For this review, take the finished solid that the model builds, in its own axes (mm). Round coordinates to 2 decimals unless told otherwise and drop trailing zeros. Order: outer loops, then holes, each group sorted by start corner. A loop starts at its lowest first (then second) coordinate and runs counter-clockwise, first axis right, second up. Notation, with made-up numbers: (32.25, 80.25) -> (53.25, 80.25) arc R20 cw to (53.25, 91.25) -> close; hole circle Ø2 at (-17.75, -9). An arc over 180 degrees is marked (long way). Put each result on its own line as item: value. Start each with the question number.
```python
from build123d import *

# Parameters (mm, degrees)
SKETCH1_W                = 80
SKETCH1_H                = 124.77
SKETCH1_R                = 5.5
BOSS_EXTRUDE1_DEPTH      = 6
F_5_0_5_DIAMETER_HOLE1_D = 5
M5X0_8_TAPPED_HOLE1_D    = 4.2
CHAMFER1_SIZE            = 2.5


with BuildPart() as part:
    # Sketch1 → Boss-Extrude1 (new body)
    with BuildSketch(Plane.XY):
        with Locations((40, 62.385)):
            Rectangle(SKETCH1_W, SKETCH1_H)
        with Locations((40, 17.57)):
            Circle(SKETCH1_R, mode=Mode.SUBTRACT)
        with BuildLine():
            Line((59.1, 94.58), (59.1, 86.58))
            ThreePointArc((59.1, 86.58), (40, 67.48), (20.9, 86.58))
            Line((20.9, 86.58), (20.9, 94.58))
            ThreePointArc((20.9, 94.58), (40, 113.68), (59.1, 94.58))
        make_face(mode=Mode.SUBTRACT)
        with BuildLine():
            Line((18.97, 118.15), (18.97, 111.15))
            ThreePointArc((18.97, 111.15), (16.43, 108.61), (13.89, 111.15))
            Line((13.89, 111.15), (13.89, 118.15))
            ThreePointArc((13.89, 118.15), (16.43, 120.69), (18.97, 118.15))
        make_face(mode=Mode.SUBTRACT)
        with BuildLine():
            Line((61.03, 118.15), (61.03, 111.15))
            ThreePointArc((61.03, 111.15), (63.57, 108.61), (66.11, 111.15))
            Line((66.11, 111.15), (66.11, 118.15))
            ThreePointArc((66.11, 118.15), (63.57, 120.69), (61.03, 118.15))
        make_face(mode=Mode.SUBTRACT)
        with BuildLine():
            Line((18.97, 63.01), (18.97, 70.01))
            ThreePointArc((18.97, 70.01), (16.43, 72.55), (13.89, 70.01))
            Line((13.89, 70.01), (13.89, 63.01))
            ThreePointArc((13.89, 63.01), (16.43, 60.47), (18.97, 63.01))
        make_face(mode=Mode.SUBTRACT)
        with BuildLine():
            Line((61.03, 63.01), (61.03, 70.01))
            ThreePointArc((61.03, 70.01), (63.57, 72.55), (66.11, 70.01))
            Line((66.11, 70.01), (66.11, 63.01))
            ThreePointArc((66.11, 63.01), (63.57, 60.47), (61.03, 63.01))
        make_face(mode=Mode.SUBTRACT)
    extrude(amount=BOSS_EXTRUDE1_DEPTH)

    # Ø5.0 (5) Diameter Hole1 (through all)
    with Locations(Plane.XY.offset(6)):
        with Locations((10.02, 20), (16.4, 41.14), (30, 40), (50, 40), (63.6, 41.14), (69.98, 20)):
            Hole(F_5_0_5_DIAMETER_HOLE1_D / 2)

    # M5x0.8 Tapped Hole1 (through all)
    with Locations(Plane.XY.offset(6)):
        with Locations((4, 120.77), (76, 120.77), (76, 4), (4, 4)):
            Hole(M5X0_8_TAPPED_HOLE1_D / 2)

    # Chamfer1
    chamfer1_edges = [part.edges().sort_by_distance(p)[0] for p in [
        (0, 124.77, 3),
        (80, 124.77, 3),
    ]]
    chamfer(chamfer1_edges, length=CHAMFER1_SIZE)


solid = part.part
```
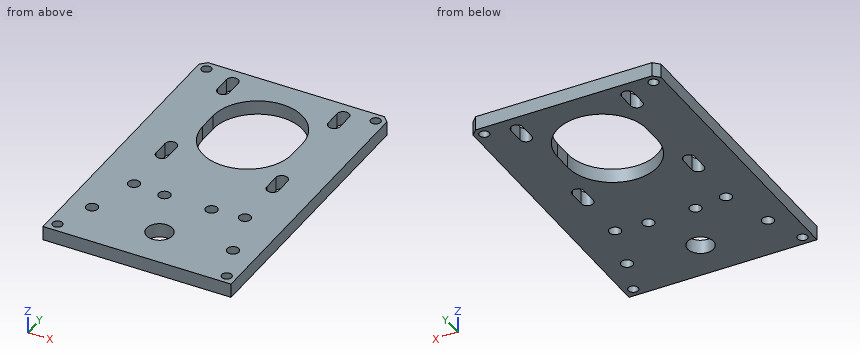
Item 1: Consider section A-A, the plane x = 40. Write out the cut boundary in (y, z).
Item 2: Consider section D-D, the plane y = 104.5. Write out the cut boundary in (x, z), plus the area to 3 significant figures.
Item 3: For L1, parallel to Y at x = 4, z = 1.3; L2, parallel to Y at x = 63.6, z = 4.3; L3, parallel to Y at x = 61.5, z = 3.7, list the stretches that pass through material, from the lowest coordinate up.
Item 4: Consider section B-B, the plane x = 10.02. Write out the cut boundary in (y, z).
Item 5: Consider section C-C, the plane y = 4. Write out the cut boundary in (x, z), plus the area to 3 significant figures.
Evaluation:
1. outline: (0, 0) -> (12.07, 0) -> (12.07, 6) -> (0, 6) -> close; (23.07, 0) -> (67.48, 0) -> (67.48, 6) -> (23.07, 6) -> close; (113.68, 0) -> (124.77, 0) -> (124.77, 6) -> (113.68, 6) -> close
2. outline: (0, 0) -> (23.68, 0) -> (23.68, 6) -> (0, 6) -> close; (56.32, 0) -> (80, 0) -> (80, 6) -> (56.32, 6) -> close
2. area: 284 mm^2
3. L1: y = 0 to 1.9, 6.1 to 118.67, 122.87 to 124.77
3. L2: y = 0 to 38.64, 43.64 to 60.47, 72.55 to 108.61, 120.69 to 124.77
3. L3: y = 0 to 39.78, 42.5 to 61.54, 71.48 to 109.68, 119.62 to 124.77
4. outline: (0, 0) -> (17.5, 0) -> (17.5, 6) -> (0, 6) -> close; (22.5, 0) -> (124.77, 0) -> (124.77, 6) -> (22.5, 6) -> close
5. outline: (0, 0) -> (1.9, 0) -> (1.9, 6) -> (0, 6) -> close; (6.1, 0) -> (73.9, 0) -> (73.9, 6) -> (6.1, 6) -> close; (78.1, 0) -> (80, 0) -> (80, 6) -> (78.1, 6) -> close
5. area: 430 mm^2
